from build123d import *

# Parameters (mm, degrees)
F1_DEPTH = 30


with BuildPart() as f1:
    # F0 (on Front) → F1 (new body)
    with BuildSketch(Plane.XZ):
        with BuildLine():
            ThreePointArc((41.6795022275, 43.1603880203), (20.2038503869, 56.496056761), (-4.8582300529, 59.8029898981))
            ThreePointArc((-4.8582300529, 59.8029898981), (-21.5105948147, 56.0115551535), (-36.4201459122, 47.6819984034))
            ThreePointArc((-36.4201459122, 47.6819984034), (-53.7829376045, 26.5969100204), (-60, 0))
            ThreePointArc((-60, 0), (-44.110621188, -40.672510353), (-4.8582300529, -59.8029898981))
            ThreePointArc((-4.8582300529, -59.8029898981), (25.3488261592, -54.382322609), (48.9239965804, -34.7338819973))
            ThreePointArc((48.9239965804, -34.7338819973), (57.1639737721, -18.2285518511), (60, 0))
            ThreePointArc((60, 0), (55.2302912071, 23.4438677094), (41.6795022275, 43.1603880203))
        make_face()
        with BuildLine():
            ThreePointArc((21.8174242293, -10), (-23.5836522276, -4.4509940021), (16.671800891, 17.2641552081))
            ThreePointArc((16.671800891, 17.2641552081), (19.5843585627, 13.8727394442), (21.8174242293, 10))
            Line((21.8174242293, 10), (34, 10))
            Line((34, 10), (34, -10))
            Line((34, -10), (21.8174242293, -10))
        make_face(mode=Mode.SUBTRACT)
        with BuildLine():
            Line((-22.4187933011, 58.3764181454), (-4.8582300529, 59.8029898981))
            ThreePointArc((-4.8582300529, 59.8029898981), (20.2038503869, 56.496056761), (41.6795022275, 43.1603880203))
            Line((41.6795022275, 43.1603880203), (78.1490666766, 80.9257275381))
            ThreePointArc((78.1490666766, 80.9257275381), (66.7614457161, 110.0684180864), (81.4361643738, 137.7022190529))
            Line((81.4361643738, 137.7022190529), (-22.4187933011, 58.3764181454))
        make_face()
        with BuildLine():
            ThreePointArc((-36.4201459122, 47.6819984034), (-21.5105948147, 56.0115551535), (-4.8582300529, 59.8029898981))
            Line((-4.8582300529, 59.8029898981), (-22.4187933011, 58.3764181454))
            Line((-22.4187933011, 58.3764181454), (-36.4201459122, 47.6819984034))
        make_face()
        with BuildLine():
            ThreePointArc((-60, 0), (-53.7829376045, 26.5969100204), (-36.4201459122, 47.6819984034))
            Line((-36.4201459122, 47.6819984034), (-22.4187933011, 58.3764181454))
            Line((-22.4187933011, 58.3764181454), (-232.5, 41.31))
            Line((-232.5, 41.31), (-232.5, 22.5))
            Line((-232.5, 22.5), (-195, 22.5))
            ThreePointArc((-195, 22.5), (-179.0900974233, 15.9099025767), (-172.5, 0))
            Line((-172.5, 0), (-60, 0))
        make_face()
        with BuildLine():
            Line((78.1490666766, 80.9257275381), (41.6795022275, 43.1603880203))
            ThreePointArc((41.6795022275, 43.1603880203), (55.2302912071, 23.4438677094), (60, 0))
            ThreePointArc((60, 0), (57.1639737721, -18.2285518511), (48.9239965804, -34.7338819973))
            Line((48.9239965804, -34.7338819973), (134.7762534316, 86.1922938025))
            ThreePointArc((134.7762534316, 86.1922938025), (107.6714265254, 70.5621088412), (78.1490666766, 80.9257275381))
        make_face()
        with BuildLine():
            ThreePointArc((-4.8582300529, -59.8029898981), (-44.110621188, -40.672510353), (-60, 0))
            Line((-60, 0), (-172.5, 0))
            ThreePointArc((-172.5, 0), (-179.0900974233, -15.9099025767), (-195, -22.5))
            Line((-195, -22.5), (-232.5, -22.5))
            Line((-232.5, -22.5), (-232.5, -41.31))
            Line((-232.5, -41.31), (-4.8582300529, -59.8029898981))
        make_face()
        with BuildLine():
            ThreePointArc((81.4361643738, 137.7022190529), (66.7614457161, 110.0684180864), (78.1490666766, 80.9257275381))
            ThreePointArc((78.1490666766, 80.9257275381), (107.6714265254, 70.5621088412), (134.7762534316, 86.1922938025))
            ThreePointArc((134.7762534316, 86.1922938025), (139.9262391764, 96.5081251439), (141.6987555688, 107.9009700508))
            ThreePointArc((141.6987555688, 107.9009700508), (120.8218243316, 141.5153060536), (81.4361643738, 137.7022190529))
        make_face()
        with BuildLine():
            ThreePointArc((119.1987555688, 107.9009700508), (110.0597224962, 94.093397249), (93.778880012, 97.1108730457))
            ThreePointArc((93.778880012, 97.1108730457), (98.3377886415, 121.7085428526), (119.1987555688, 107.9009700508))
        make_face(mode=Mode.SUBTRACT)
    extrude(amount=F1_DEPTH)


solid = f1.part
Geometry: final body of the model. Coordinates: model frame, mm. A direction names the side the tool comes from. Round coordinates to 2 decimals unless told otherwise and drop trailing zeros. Write each loop counter-clockwise with the first axis right and the second up, starting at its lowest first coordinate (ties: lowest second). Pieces come first, ordered by that corner, then holes. Notation, with made-up numbers: M 2.25,-24 L 25.25,-24 A24 cw 25.25,8 Z; hole C 51,31 d10. An arc over 180 degrees is marked long. Write item = value, one per line.
Item 1: Section query A-A on x = -204. Return loops of the section in (y, z).
Findings:
outline = M -30,-43.63 L 0,-43.63 L 0,-22.5 L -30,-22.5 Z; M -30,22.5 L 0,22.5 L 0,43.63 L -30,43.63 Z
Item 2: Material intervals for line 1 along Z through (x, y) = (11, -18.75); line 2 along Z through (x, y) = (-194, -7.75); line 3 along X through (y, z) = (-24, -10.5), sorted ascending. Write a range as [from, to].
Findings:
line_1 = [-58.98, -21.33], [21.33, 83.9]
line_2 = [-44.44, -22.48], [22.48, 44.44]
line_3 = [-175.1, -21.58], [21.58, 66.13]
Item 3: Section query B-B on y = -4. Return loops of the section in (x, z), then the cut area to 3 significant figures.
Findings:
outline = M -232.5,-41.31 L -4.86,-59.8 A60 ccw 48.92,-34.73 L 134.78,86.19 A37.5 ccw 81.44,137.7 L -22.42,58.38 L -232.5,41.31 L -232.5,22.5 L -195,22.5 A22.5 cw -195,-22.5 L -232.5,-22.5 Z; hole M 21.82,-10 L 34,-10 L 34,10 L 21.82,10 A24 ccw long Z; hole C 104.2,107.9 d30
area = 35,400 mm^2
Item 4: Access query for faces 4 (the face through (-232.5, -15, 32)), 5 (the face through (28, -15, -10)), 6 (the face through (-214, -15, 22.5)). Directions: +Z, -Z, +X, -X, +Y, -Y. A direction counts if a zero-diameter tool reaches every point of the face in a straight line with its end or side. Return the directions, or none.
Findings:
face_4 = +Z, -Z, -X, +Y, -Y
face_5 = +Y, -Y
face_6 = -X, +Y, -Y
Item 5: Section query D-D on z = 63. Return loops of the section in (x, y), then the cut area to 3 significant figures.
Findings:
outline = M -16.37,-30 L 118.31,-30 L 118.31,0 L -16.37,0 Z
area = 4,040 mm^2
Item 6: Pin query (flat end, axial travel): P1, Ø8, axis at y = -23.5, z = 91, coming from the -X side; P2, Ø10, axis at x = -162, z = 36.5, coming from the +Y side; P3, Ø3, axis at y = -16, z = -10.5, coming from the +X side; P4, Ø6, axis at x = 29.5, y = -18.5, coming from the +Z side. Return the tip coordinate at first contact, or that it passes through.
Findings:
P1 = 15.06
P2 = 0
P3 = 67.19
P4 = 100.32
Item 7: Pull-direction query (Z, two-part tool) for faces 1 (the face through (-125.989, -14.79, 49.963)), 2 (the face through (-172.505, -14.79, 0.495)), 3 (the face through (24.954, -14.79, -54.564)); classes: pulls with the +Z half, pulls with the -Z half, needs draft (parallel to the pull), parting line crosses it, or undercut.
Findings:
face_1 = pulls with the +Z half
face_2 = undercut
face_3 = pulls with the -Z half
Item 8: Section query C-C on z = 0. Return loops of the section in (x, y).
Findings:
outline = M -172.5,-30 L -24,-30 L -24,0 L -172.5,0 Z; M 34,-30 L 73.58,-30 L 73.58,0 L 34,0 Z
